The figure shows three views and two pictorial views of one solid part (mm, origin at its lowest corner). Answer the questions. A direction names the side the tool comes from. Round coordinates to 2 decimals unless told otherwise and drop trailing zeros. Order: outer loops, then holes, each group sorted by start corner. A loop starts at its lowest first (then second) coordinate and runs counter-clockwise, first axis right, second up. Notation, with made-up numbers: (-19, 48) -> (22, 48) arc R17 cw to (22, 69) -> close; hole circle Ø3 at (82, -27.5). An arc over 180 degrees is marked (long way). Return JSON: item names as keys, results as strings. Group by question number.
(1) Consider line 1 (Z direction, x = 13, y = 14.5); line 2 (X direction, y = 39, z = 74) (1 decimal); line 3 (Y direction, x = 14, z = 68). Determine where each line is inside the solid, lowest interval first. Write a range as [from, to].
(2) The part is cut by section C-C (z = 17). Determine the outline of the cut face in (x, y) (1 decimal).
(3) Determine the mould class of the marked faces 1, 2 and 3 for opening direction Y: +Y half, -Y half, draft (parallel to the pull), parting line (faces both ways), or undercut.
(4) Each of these flat-tipped pins is pushed along its axis until it touches: pin 1 (6 mm diameter, centred on y = 42.5, z = 21, fed in from +X); pin 2 (12 mm diameter, centred on x = 30, z = 10.5, fed in from +Y); pin 3 (10 mm diameter, centred on x = 52.5, y = 57.5, fed in from -Z). Where does it stop, or does it pass through?
(5) The part is cut by section A-A (x = 24). Determine the outline of the cut face in (y, z).
(6) Which of the six approach directions +Z, -Z, +X, -X, +Y, -Y give full straight-line access (tool end or side, diameter ignored) to the marked faces 4 and 5?
(7) The part is cut by section D-D (x = 33). Determine the outline of the cut face in (y, z) (1 decimal), plus the area to 3 significant figures.
(8) The part is cut by section B-B (y = 27). Determine the outline of the cut face in (x, z).
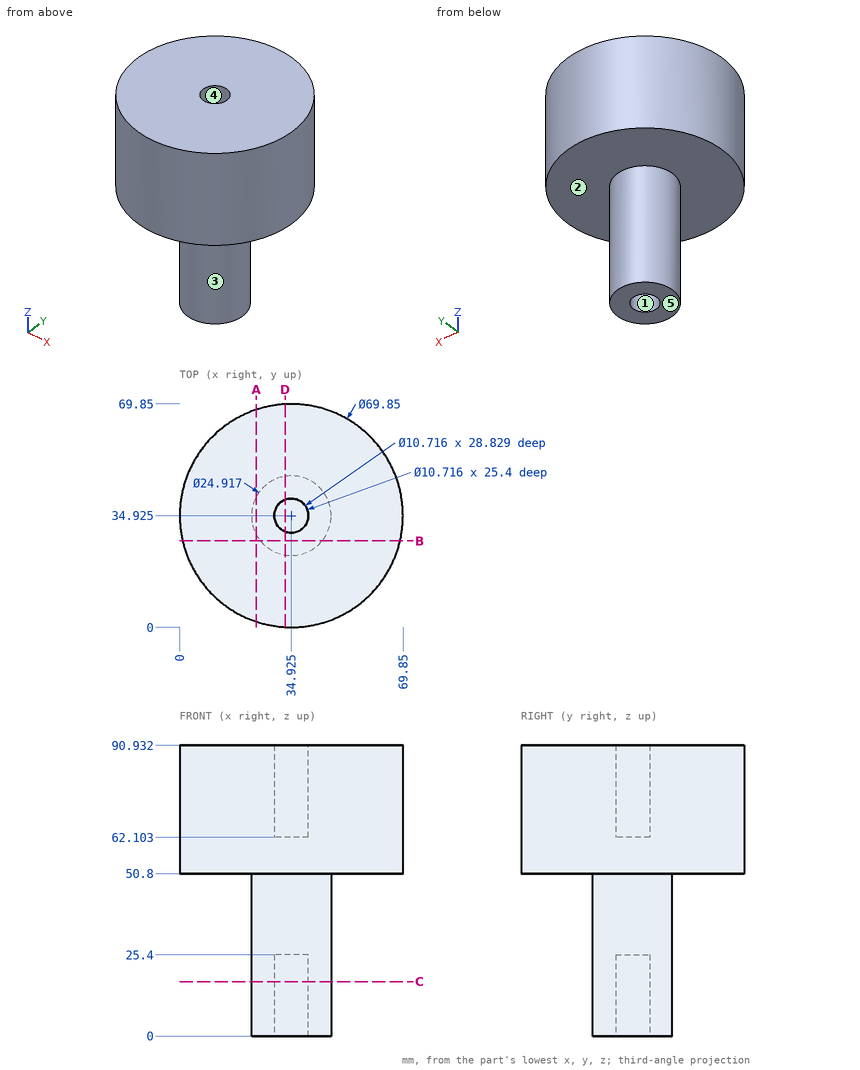
Answer below:
{
 "1": {"line 1": "z = [50.8, 90.93]", "line 2": "x = [0.2, 31.4], [38.4, 69.6]", "line 3": "y = [6.96, 62.89]"},
 "2": {"outline": "circle Ø24.9 at (34.9, 34.9); hole circle Ø10.7 at (34.9, 34.9)"},
 "3": {"face 1": "undercut", "face 2": "draft", "face 3": "parting line"},
 "4": {"pin 1": "stops at x = 46.51", "pin 2": "stops at y = 47.38", "pin 3": "stops at z = 50.8"},
 "5": {"outline": "(1.75, 50.8) -> (28.94, 50.8) -> (28.94, 0) -> (40.91, 0) -> (40.91, 50.8) -> (68.1, 50.8) -> (68.1, 90.93) -> (1.75, 90.93) -> close"},
 "6": {"face 4": "+Z", "face 5": "-Z, +X, -X, +Y, -Y"},
 "7": {"outline": "(0.1, 50.8) -> (22.6, 50.8) -> (22.6, 0) -> (29.9, 0) -> (29.9, 25.4) -> (39.9, 25.4) -> (39.9, 0) -> (47.2, 0) -> (47.2, 50.8) -> (69.8, 50.8) -> (69.8, 90.9) -> (39.9, 90.9) -> (39.9, 62.1) -> (29.9, 62.1) -> (29.9, 90.9) -> (0.1, 90.9) -> close", "area": "3,510 mm²"},
 "8": {"outline": "(0.91, 50.8) -> (25.31, 50.8) -> (25.31, 0) -> (44.54, 0) -> (44.54, 50.8) -> (68.94, 50.8) -> (68.94, 90.93) -> (0.91, 90.93) -> close"}
}
